from build123d import *

# Parameters (mm, degrees)
BOSS_EXTRUDE1_REACH = 66.721
SKETCH3_W           = 64.787323871
SKETCH3_H           = 20.939874787


with BuildPart() as part:
    # Sketch1 → Revolve1 (revolve)
    with BuildSketch(Plane.XY):
        with BuildLine():
            Line((19, 74.817317551), (21, 74.817317551))
            Line((21, 74.817317551), (21, 87.817317551))
            Line((21, 87.817317551), (29, 87.817317551))
            Line((29, 87.817317551), (29, 84.817317551))
            Line((29, 84.817317551), (48.884927091, 84.817317551))
            Line((48.884927091, 84.817317551), (48.884927091, 79.817317551))
            Line((48.884927091, 79.817317551), (37.26232647, 79.817317551))
            add(Edge.make_bspline(
                [(37.26232647, 79.817317551), (35.317542772, 79.817317551), (31.576426132, 78.956130843), (28.504834315, 74.722950853), (26.811531328, 69.225059311), (27.023440035, 67.0117878), (26.529376961, 61.457439784), (26.110101007, 49.682029535)],
                knots=[0, 0, 0, 0, 0.027814375, 0.048077406, 0.056130992, 0.108350232, 0.258095951, 0.258095951, 0.258095951, 0.258095951], degree=3))
            Line((26.110101007, 49.682029535), (25.002372474, 18.571354555))
            add(Edge.make_bspline(
                [(64.528129231, -17.987011239), (65.304995671, -15.790991926), (62.495595706, -12.403296178), (55.378812109, -12.037399906), (46.505259928, -12.035031844), (35.990414113, -11.165636172), (27.978614985, -4.711317004), (25.439837988, 5.526983198), (24.863232294, 14.663587636), (25.002372474, 18.571354555)],
                knots=[0, 0, 0, 0, 0.097399991, 0.161218221, 0.32460028, 0.514717464, 0.634012286, 0.770814213, 1, 1, 1, 1], degree=3))
            Line((64.528129231, -17.987011239), (47, -17.987011239))
            Line((47, -17.987011239), (47, -38.859991473))
            Line((47, -38.859991473), (35.75, -38.859991473))
            Line((35.75, -38.859991473), (35.75, -59.79986626))
            Line((35.75, -59.79986626), (33.434340492, -59.79986626))
            Line((33.434340492, -59.79986626), (31.360417848, -39.321612307))
            Line((31.360417848, -39.321612307), (31.360417848, -34.480558786))
            Line((31.360417848, -34.480558786), (17.5, -34.480558786))
            Line((17.5, -34.480558786), (17.5, -23.480558786))
            Line((17.5, -23.480558786), (15.5, -23.480558786))
            Line((15.5, -23.480558786), (19, 74.817317551))
        make_face()
    revolve(axis=Axis((0, 926.027727684, 0), (0, -1, 0)))

    # Sketch3 → Boss-Extrude1 (add, up to next)
    with BuildSketch(Plane(origin=(0, 0, 0), x_dir=(0, 0, -1), z_dir=(1, 0, 0)), mode=Mode.PRIVATE) as boss_extrude1_sk1:
        with Locations((-0.273634545, -49.329928866)):
            Rectangle(SKETCH3_W, SKETCH3_H)
    boss_extrude1_tool1 = extrude(boss_extrude1_sk1.sketch, amount=BOSS_EXTRUDE1_REACH, mode=Mode.PRIVATE) - part.part
    add(boss_extrude1_tool1.solids().sort_by_distance((0, -49.329929, 0.273635))[0])


solid = part.part
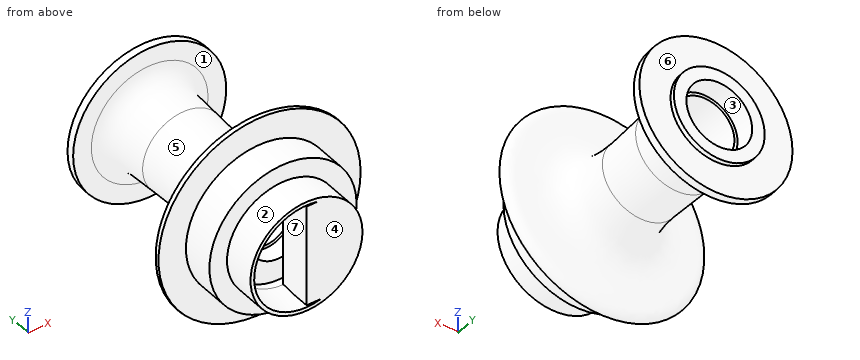
Here's how the part is built. I have some questions about the finished solid (model axes, mm). Face numbers are marked on the shaded views. A direction names the side the tool comes from. Give positions to 0.01 mm unless a question says otherwise; leave off trailing zeros. Loops run counter-clockwise (first coordinate to the right, second up) from the corner with the lowest first, then second, coordinate; pieces in that order, holes last. Notation, with made-up numbers: (-6, 5.5) -> (3, 5.5) arc R15 ccw to (3, 20.5) -> close; hole circle Ø6 at (7, 84.5). An arc over 180 degrees is marked (long way). One line per item, written item: value.
Q1. We'd pull the mould along Y, two halves only. Please class the marked faces 4, 5, 6 and 7: pulls with the +Y half, pulls with the -Y half, needs draft (parallel to the pull), parting line crosses it, or undercut.
Answers follow:
face 4: pulls with the -Y half
face 5: undercut
face 6: pulls with the +Y half
face 7: needs draft
Q2. Suppose I cut it at A-A on y = 47.5. Please give me the cut outline in (x, z).
Answers follow:
outline: circle Ø52.06 at (0, 0); hole circle Ø36.05 at (0, 0)
Q3. I'm going to push flat-ended pins straight in: pin 1 Ø8 at (x, z) = (26.5, 35.5) entering from +Y; pin 2 Ø10 at (x, y) = (4.5, -56.5) entering from -Z; pin 3 Ø9.5 at (x, z) = (8, 1.5) entering from +Y. Where does each tip first touch, or does it pass through?
Answers follow:
pin 1: y = 84.82
pin 2: z = -35.75
pin 3: y = -38.86
Q4. On a 3-axis mill with a long thin cutter (end or side, diameter ignored), from which of +Z, -Z, +X, -X, +Y, -Y can I reach the whole of each face in a straight line? I mean the marked faces 1, 2 and 3. Say none if no direction works.
Answers follow:
face 1: none
face 2: -Y
face 3: +Y
Q5. If I drill on line 1 along Z through (x, y) = (0, -29); line 2 along Y through (x, z) = (36, -24); line 3 along Z through (x, y) = (1, 45), over which ranges is the centre line in solid material (lowest first)?
Answers follow:
line 1: -47 to -17.5, 17.5 to 47
line 2: -38.86 to -11.66, 79.82 to 84.82
line 3: -25.92 to -17.91, 17.91 to 25.92
